Autodesk Inventor part; units mm, degrees
ref_plane "YZ Plane" through (0, 0, 0) normal (1, 0, 0) x (0, 1, 0)
ref_plane "XZ Plane" through (0, 0, 0) normal (0, 1, 0) x (-1, 0, 0)
ref_plane "XY Plane" through (0, 0, 0) normal (0, 0, 1) x (1, 0, 0)
sketch "Szkic1" plane through (0, 0, 0) normal (0, 0, 1) x (1, 0, 0)
  line L0 (-25.3316, -15.5729) -> (26.0684, -15.5729)
  line L1 (26.0684, -15.5729) -> (26.0684, 35.4271)
  line L2 (26.0684, 35.4271) -> (26.0684, 35.4271)
  line L3 (26.0684, 35.4271) -> (26.0684, 55.4271)
  line L4 (26.0684, 55.4271) -> (-5.3316, 55.4271)
  line L5 (-5.3316, 55.4271) -> (-5.3316, 86.8271)
  line L6 (-5.3316, 86.8271) -> (-25.3316, 86.8271)
  line L7 (-25.3316, -15.5729) -> (-25.3316, 86.8271)
  line L8 (-15.6316, 16.9271) -> (16.3684, 16.9271)
  line L9 (16.3684, 16.9271) -> (16.3684, -15.0729)
  line L10 (16.3684, -15.0729) -> (-15.6316, -15.0729)
  line L11 (-15.6316, -15.0729) -> (-15.6316, 16.9271)
  circle A0 centre (0.3684, 0.9271) radius 11
  circle A1 centre (0.3684, 0.9271) radius 16
  line L12 (-25.3316, 51.9271) -> (-96.8316, 51.9271)
  line L13 (-96.8316, 51.9271) -> (-96.8316, 36.9271)
  line L14 (-96.8316, 36.9271) -> (-25.3316, 36.9271)
  line L15 (-25.3316, 36.9271) -> (-25.3316, 51.9271)
  point P0 (0, 0)
  point P1 (-10.9453, 12.2408)
  point P2 (11.6821, 12.2408)
  point P3 (11.6821, -10.3866)
  point P4 (-10.9453, -10.3866)
  point P5 (16.0684, 45.4271)
  point P6 (-15.3316, 76.8271)
  point P7 (-15.3316, 45.4271)
  point P8 (-91.8316, 44.4271)
  point P9 (-75.8316, 44.4271)
  dimension "d0" = 20
  dimension "d1" = 20
  dimension "d2" = 51.4
  dimension "d3" = 51.4
  dimension "d4" = 34.5
  dimension "d5" = 25.7
  dimension "d6" = 51.4
  dimension "d7" = 51
  dimension "d8" = 32
  dimension "d9" = 32
  dimension "d10" = 16
  dimension "d11" = 16
  dimension "d12" = 22
  dimension "d13" = 32
  dimension "d23" = 10
  dimension "d24" = 10
  dimension "d25" = 10
  dimension "d26" = 10
  dimension "d27" = 10
  dimension "d28" = 10
  dimension "d45" = 71.5
  dimension "d46" = 15
  dimension "d47" = 18.5
  dimension "d57" = 5
  dimension "d58" = 16
  dimension "d59" = 7.5
  dimension "d60" = 7.5
extrude "Wyciągnięcie proste1" add sketch "Szkic1" along normal blind 4 contours L7 L6 L5 L4 L3 L1 L0 | L8 A1 L11 | L8 L9 A1 | A1 | A1 L10 L11 | L9 L10 A1
hole "Otwór1" at (0.3684, 0.9271, 0) at (-10.9453, 12.2408, 0) at (11.6821, 12.2408, 0) at (11.6821, -10.3866, 0) at (-10.9453, -10.3866, 0) direction (0, 0, 1) diameter 4 end through all
hole "Otwór2" at (16.0684, 45.4271, 0) at (-15.3316, 76.8271, 0) at (-15.3316, 45.4271, 0) direction (0, 0, 1) diameter 4 end through all
chamfer "Faza1" distance 51 distance2 9.7 1 edges at (-25.3316, -15.5729, 2) measured on face at (-25.3316, 18.5605, 1.3333)
chamfer "Faza2" distance 51 distance2 9.7 1 edges at (26.0684, -15.5729, 2) measured on face at (26.0684, 31.7605, 1.3333)
fillet "Zaokrąglenie1" radius 2 2 edges at (-15.6316, -15.5729, 2) (16.3684, -15.5729, 2)
fillet "Zaokrąglenie2" radius 6 4 edges at (-5.3316, 55.4271, 2) (26.0684, 55.4271, 2) (-5.3316, 86.8271, 2) (-25.3316, 86.8271, 2)
extrude "Wyciągnięcie proste2" add sketch "Szkic1" along normal blind 4 contours L14 L13 L12 L7
chamfer "Faza3" distance 8 distance2 45.5 1 edges at (-25.3316, 51.9271, 2) measured on face at (-25.3316, 61.5605, 1.3333)
fillet "Zaokrąglenie4" radius 10 2 edges at (-25.3316, 59.9271, 2) (-25.3316, 36.9271, 2)
chamfer "Faza4" distance 2 angle 45 1 edges at (-96.8316, 36.9271, 2)
hole "Otwór3" at (-91.8316, 44.4271, 0) at (-75.8316, 44.4271, 0) direction (0, 0, 1) diameter 3 end through all
equation "\"d1\" = d0"
equation "\"d2\" = d6"
equation "\"d3\" = d6"
equation "\"d6\" = 2 * d5"
properties part number "LC_ALU_4mm_Heatbed_Frame_Linear_Bearing_Mounting_Bracket_Cable_Chain"
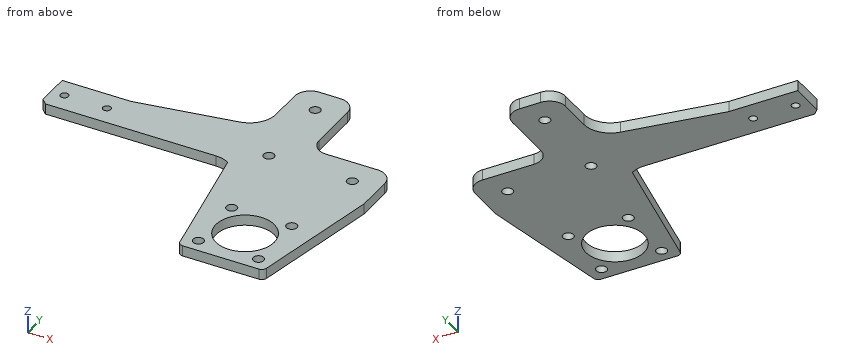
Read the model definition and answer for the solid it produces. Units are mm, in the model's axes. Coordinates: 2 decimals unless noted, no trailing zeros. Order: outer loops, then holes, each group sorted by start corner. A loop starts at its lowest first (then second) coordinate and runs counter-clockwise, first axis right, second up. Notation, with made-up numbers: M 4.5,-14.5 L 20.5,-14.5 A13 ccw 20.5,8.5 Z; hole C -9.5,17 d4. An arc over 180 degrees is marked long. Put each result on its own line as item: value. Start each with the question number.
Item 1: Section A-A, the plane y = 76.5 is taken. Determine the outline of the cut face in (x, z), plus the area to 3 significant figures.
Item 2: Consider probe 1 along X at (y, z) = (10.5, 1.3); probe 2 along Y at (x, z) = (10.5, 2.9); probe 3 along Y at (x, z) = (-8.5, 2.25). Determine where each line is inside the solid, lowest interval first. Write a range as [from, to].
Item 3: Given pin 1 Ø2 at (y, z) = (68.5, 2.5) entering from +X; pin 2 Ø1.2 at (x, z) = (-86, 2.5) entering from +Y; pin 3 Ø1.5 at (y, z) = (28, 3) entering from -X, each flat-ended and moving along its own axis, determine where each tip first touches the part or whether it passes through.
Item 4: Section B-B, the plane x = -7.5 is taken. Determine the outline of the cut face in (y, z), plus the area to 3 significant figures.
Item 5: Section D-D, the plane x = -83.5 is taken. Determine the outline of the cut face in (y, z).
Item 6: Section C-C, the plane z = 0.65 is taken. Count the separate pieces of the cut face and the enclosed holes in it, plus the area to 3 significant figures.
Computed:
1. outline: M -25.33,0 L -17.3,0 L -17.3,4 L -25.33,4 Z; M -13.36,0 L -5.33,0 L -5.33,4 L -13.36,4 Z
1. area: 64.2 mm2
2. probe 1: x = [-20.59, -11.93], [-9.96, -5.05], [5.79, 10.7], [12.67, 21.33]
2. probe 2: y = [-15.57, -12], [-8.77, -3.36], [5.21, 10.63], [13.85, 55.43]
2. probe 3: y = [-15.57, -5.58], [7.43, 86.12]
3. pin 1: stops at x = -5.33
3. pin 2: stops at y = 51.93
3. pin 3: stops at x = -24.06
4. outline: M -15.57,0 L -6.76,0 L -6.76,4 L -15.57,4 Z; M 8.61,0 L 85.44,0 L 85.44,4 L 8.61,4 Z
4. area: 343 mm2
5. outline: M 36.93,0 L 51.93,0 L 51.93,4 L 36.93,4 Z
6. separate pieces: 1
6. enclosed holes: 10
6. area: 4,550 mm2
